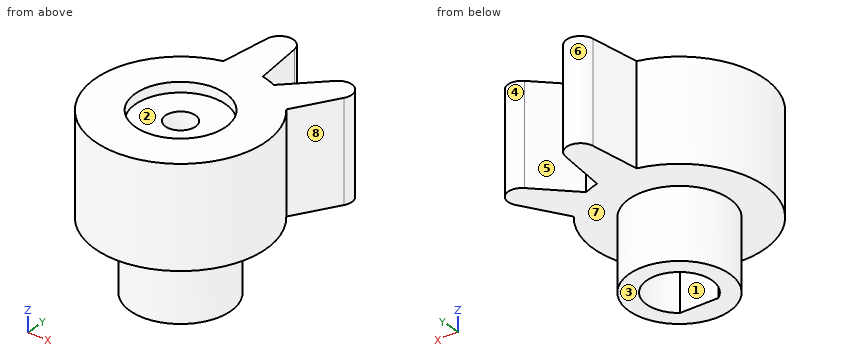
from build123d import *

# Parameters (mm, degrees)
SKETCH1_R           = 1.5
BOSS_EXTRUDE1_DEPTH = 10
SKETCH5_R           = 5
BOSS_EXTRUDE3_DEPTH = 7
SKETCH8_R           = 4.5
CUT_EXTRUDE2_DEPTH  = 1


with BuildPart() as part:
    # Sketch1 → Boss-Extrude1 (new body)
    with BuildSketch(Plane.XY):
        with BuildLine():
            Line((-1.390653283, 13.224086579), (-2, 8.261355821))
            ThreePointArc((-2, 8.261355821), (-2.767329313, -8.036907893), (6.66222002, 5.278714276))
            Line((6.66222002, 5.278714276), (9.237410395, 9.564550779))
            ThreePointArc((9.237410395, 9.564550779), (8.899037344, 11.390248383), (7.045710912, 11.276894083))
            Line((7.045710912, 11.276894083), (3.510177006, 7.741360177))
            ThreePointArc((3.510177006, 7.741360177), (2.767329313, 8.036907893), (2, 8.261355821))
            Line((2, 8.261355821), (1.390653283, 13.224086579))
            ThreePointArc((1.390653283, 13.224086579), (0, 14.454432673), (-1.390653283, 13.224086579))
        make_face()
        Circle(SKETCH1_R, mode=Mode.SUBTRACT)
    extrude(amount=BOSS_EXTRUDE1_DEPTH)

    # Sketch5 → Boss-Extrude3 (add)
    with BuildSketch(Plane(origin=(0, 0, 0), x_dir=(-1, 0, 0), z_dir=(0, 0, -1))):
        with Locations(Location((0, 0, 0), (0, 0, 180))):
            Circle(SKETCH5_R)
        with BuildLine():
            Line((1.95, -2.6), (-1.95, -2.6))
            ThreePointArc((-1.95, -2.6), (0, 3.25), (1.95, -2.6))
        make_face(mode=Mode.SUBTRACT)
    extrude(amount=BOSS_EXTRUDE3_DEPTH)

    # Sketch8 → Cut-Extrude2 (cut)
    with BuildSketch(Plane.XY.offset(10)):
        Circle(SKETCH8_R)
    extrude(amount=-CUT_EXTRUDE2_DEPTH, mode=Mode.SUBTRACT)


solid = part.part
Design review of the part built by this model. Coordinates are the model's own, in mm. Face numbers are marked on the shaded views. A direction names the side the tool comes from. Coordinates: 2 decimals unless noted, no trailing zeros. Write each loop counter-clockwise with the first axis right and the second up, starting at its lowest first coordinate (ties: lowest second). Pieces come first, ordered by that corner, then holes. Notation, with made-up numbers: (70.25, 41) - (129.25, 41) arc R18 cw to (129.25, 75) - close; hole circle Ø7 at (80.5, -5). An arc over 180 degrees is marked (long way). One line per item, written item: value.
1) Add section A-A (x = 0). State the section outline as (y, z) points.
Answer sheet:
outline: (-8.5, 0) - (-5, 0) - (-5, -7) - (-2.6, -7) - (-2.6, 0) - (-1.5, 0) - (-1.5, 9) - (-4.5, 9) - (-4.5, 10) - (-8.5, 10) - close; (1.5, 0) - (3.25, 0) - (3.25, -7) - (5, -7) - (5, 0) - (14.45, 0) - (14.45, 10) - (4.5, 10) - (4.5, 9) - (1.5, 9) - close
2) Mouldability with a two-part tool opening along Y and no side actions: class the marked faces 6, 7 and 8 as +Y half, -Y half, draft (parallel to the pull), parting line (faces both ways), or undercut.
Answer sheet:
face 6: +Y half
face 7: draft
face 8: undercut
3) Add section C-C (y = 1). State the section outline as (x, z) points.
Answer sheet:
outline: (-8.44, 0) - (-4.9, 0) - (-4.9, -7) - (-3.09, -7) - (-3.09, 0) - (-1.12, 0) - (-1.12, 9) - (-4.39, 9) - (-4.39, 10) - (-8.44, 10) - close; (1.12, 0) - (3.09, 0) - (3.09, -7) - (4.9, -7) - (4.9, 0) - (8.44, 0) - (8.44, 10) - (4.39, 10) - (4.39, 9) - (1.12, 9) - close
4) Add section D-D (y = -2.25). State the section outline as (x, z) points, plus the area to 3 significant figures.
Answer sheet:
outline: (-8.2, 0) - (-4.47, 0) - (-4.47, -7) - (-2.35, -7) - (-2.35, 0) - (2.35, 0) - (2.35, -7) - (4.47, -7) - (4.47, 0) - (8.2, 0) - (8.2, 10) - (3.9, 10) - (3.9, 9) - (-3.9, 9) - (-3.9, 10) - (-8.2, 10) - close
area: 186 mm2
5) Insertion check: pin 1 (8.5 mm diameter, centred on x = 0, y = 0, fed in from +Z); pin 2 (6 mm diameter, centred on y = 2, z = 8, fed in from +X); pin 3 (8 mm diameter, centred on y = -6, z = -3, fed in from -X). Each pin has a flat end and moves straight along its axis. Give the tip position at first contact, or say it passes through.
Answer sheet:
pin 1: stops at z = 9
pin 2: stops at x = 8.5
pin 3: stops at x = -7.81
6) For the marked faces 1, 2, 3, 4 and 5, list the 3-axis set-ups (+Z, -Z, +X, -X, +Y, -Y) from which the entire face can be reached by the end or side of a thin tool; tool diameter is ignored.
Answer sheet:
face 1: -Z
face 2: +Z
face 3: -Z, +X, -X, +Y, -Y
face 4: +Z, -Z
face 5: +Z, -Z, +Y
7) To check wall thickness, follow probe 1 along Y at (x, z) = (0, 9.5); probe 2 along Y at (x, z) = (0, 3.75); probe 3 along Z at (x, y) = (2.75, -2.5). State the ranges of each line that lie inside material, in increasing order.
Answer sheet:
probe 1: y = -8.5 to -4.5, 4.5 to 14.45
probe 2: y = -8.5 to -1.5, 1.5 to 14.45
probe 3: z = -7 to 9
8) Add section B-B (z = 1). State the section outline as (x, y) points.
Answer sheet:
outline: (-2, 8.26) arc R8.5 ccw (long way) to (6.66, 5.28) - (9.24, 9.56) arc R1.4 ccw to (7.05, 11.28) - (3.51, 7.74) arc R8.5 ccw to (2, 8.26) - (1.39, 13.22) arc R1.4 ccw to (-1.39, 13.22) - close; hole circle Ø3 at (0, 0)
